Here's how the part is built. I have some questions about the finished solid (model axes, mm). A direction names the side the tool comes from. Give positions to 0.01 mm unless a question says otherwise; leave off trailing zeros. Write each loop counter-clockwise with the first axis right and the second up, starting at its lowest first coordinate (ties: lowest second). Pieces come first, ordered by that corner, then holes. Notation, with made-up numbers: (58, 30.25) - (62, 30.25) arc R31 ccw to (62, 68.25) - close; hole circle Ø9 at (35.5, 35). An arc over 180 degrees is marked (long way). One line per item, written item: value. Start each with the question number.
1) Imagine slicing it at A-A on x = 1.5. Write out the boundary of the cut face in (y, z).
2) Please list where these lines run through material, in increasing order: L1, parallel to Y at x = 5.75, z = 0; L2, parallel to X at y = 5, z = 3; L3, parallel to Z at x = 4, y = -0.75. Write a range as [from, to].
3) I'm going to push flat-ended pins straight in: P1, Ø12, axis at y = 4, z = -7, coming from the -X side; P2, Ø2, axis at x = 1.5, z = 4.5, coming from the +Y side; P3, Ø1.5, axis at x = 5, z = 1.5, coming from the -Y side. Where does each tip first touch, or does it pass through?
4) We'd pull the mould along Z, two halves only. Please class faces 4 (the flat face through (7, -10, -2)), 5 (the cylindrical face through (0.62, -8.43, 4.38)): +Z half, -Z half, draft (parallel to the pull), parting line (faces both ways), or undercut.
5) On a 3-axis mill with a long thin cutter (end or side, diameter ignored), from which of +Z, -Z, +X, -X, +Y, -Y can I reach the whole of each face in a straight line? I mean faces 1 (the flat face through (0, -4, -2)), 2 (the cylindrical face through (6.38, 9.274, -2.059)), 3 (the flat face through (1, -4, 4)). Say none if no direction works.
from build123d import *

# Parameters (mm, degrees)
SKETCH1_R          = 11
SKETCH1_R_2        = 4
EXTRUDE1_DEPTH     = 7
CHAMFER1_SIZE      = 0.25
SKETCH2_R          = 9.5
SKETCH2_R_2        = 5.5
CUT_EXTRUDE1_DEPTH = 1
SKETCH3_R          = 9.5
SKETCH3_R_2        = 5.5
CUT_EXTRUDE2_DEPTH = 1
CHAMFER2_SIZE      = 0.25


with BuildPart() as part:
    # Sketch1 → Extrude1 (new body)
    with BuildSketch(Plane(origin=(0, 0, 0), x_dir=(0, 0, -1), z_dir=(1, 0, 0))):
        Circle(SKETCH1_R)
        Circle(SKETCH1_R_2, mode=Mode.SUBTRACT)
    extrude(amount=EXTRUDE1_DEPTH)

    # Chamfer1
    chamfer1_edges = [part.edges().sort_by_distance(p)[0] for p in [
        (0, 0, 11),
        (7, 0, 11),
        (0, 0, 4),
    ]]
    chamfer(chamfer1_edges, length=CHAMFER1_SIZE)

    # Sketch2 → Cut-Extrude1 (cut)
    with BuildSketch(Plane.ZY):
        Circle(SKETCH2_R)
        Circle(SKETCH2_R_2, mode=Mode.SUBTRACT)
    extrude(amount=-CUT_EXTRUDE1_DEPTH, mode=Mode.SUBTRACT)

    # Sketch3 → Cut-Extrude2 (cut)
    with BuildSketch(Plane(origin=(7, 0, 0), x_dir=(0, 0, -1), z_dir=(1, 0, 0))):
        with Locations(Location((0, 0, 0), (0, 0, 180))):  # turned: the seam where the file's is
            Circle(SKETCH3_R)
        with Locations(Location((0, 0, 0), (0, 0, 180))):  # turned: the seam where the file's is
            Circle(SKETCH3_R_2, mode=Mode.SUBTRACT)
    extrude(amount=-CUT_EXTRUDE2_DEPTH, mode=Mode.SUBTRACT)

    # Chamfer2
    chamfer2_edges = [part.edges().sort_by_distance(p)[0] for p in [
        (0, 0, -9.5),
        (0, 0, -5.5),
        (7, 0, -9.5),
        (7, 0, -5.5),
    ]]
    chamfer(chamfer2_edges, length=CHAMFER2_SIZE)


solid = part.part
Numbers:
1. outline: circle Ø22 at (0, 0); hole circle Ø8 at (0, 0)
2. L1: [-11, -4], [4, 11]
2. L2: [1, 6]
2. L3: [-10.97, -3.93], [3.93, 10.97]
3. P1: x = 0
3. P2: y = 10.43
3. P3: y = -10.97
4. face 4: draft
4. face 5: undercut
5. face 1: +Z, -Z, -X, +Y, -Y
5. face 2: +X
5. face 3: -X
